from build123d import *


with BuildPart() as part:
    # Sketch2 → Revolve1 (revolve)
    with BuildSketch(Plane.XY, mode=Mode.PRIVATE) as revolve1_sk:
        with BuildLine():
            Line((7.900124766, 45.904993762), (46, 44))
            Line((46, 44), (46, 40))
            Line((46, 40), (8, 40))
            ThreePointArc((8, 40), (6.585786438, 39.414213562), (6, 38))
            Line((6, 38), (6, 2))
            Line((6, 2), (0, 2))
            Line((0, 2), (0, 76.2))
            Line((0, 76.2), (6.299212598, 76.2))
            Line((6.299212598, 76.2), (100, 76.2))
            Line((100, 76.2), (100, 73.2))
            Line((100, 73.2), (8, 73.2))
            ThreePointArc((8, 73.2), (6.585786438, 72.614213562), (6, 71.2))
            Line((6, 71.2), (6, 47.902498439))
            ThreePointArc((6, 47.902498439), (6.550905374, 46.524048308), (7.900124766, 45.904993762))
        make_face()
    revolve(revolve1_sk.sketch.rotate(Axis((0, 0, 0), (1, 0, 0)), 90), axis=Axis((0, 0, 0), (1, 0, 0)))


solid = part.part
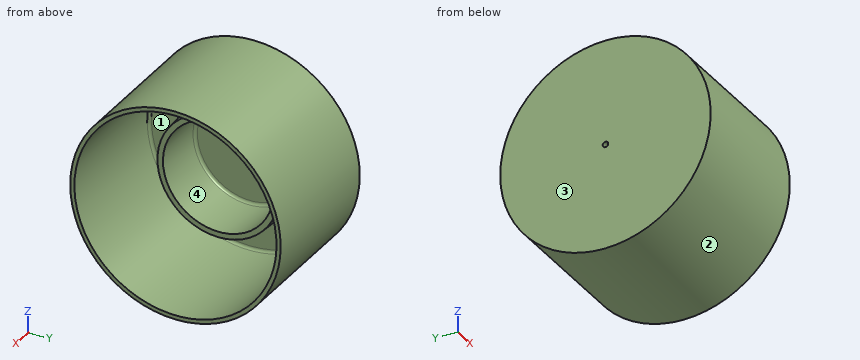
Input: part model. Units: mm. Frame: model coordinates. Face numbers are marked on the shaded views. Give positions to 0.01 mm unless a question says otherwise; leave off trailing zeros. Order: outer loops, then holes, each group sorted by start corner. A loop starts at its lowest first (then second) coordinate and runs counter-clockwise, first axis right, second up. Notation, with made-up numbers: M 80,14.5 L 128,14.5 A37 ccw 128,50.5 Z; hole C 62.25,9.25 d3. An arc over 180 degrees is marked long. Answer as a JSON object with one key per item and string values.
1. Cut plane B-B, the plane x = 22. Output: boundary loops of the cut face in (y, z).
Result sheet:
{"outline": "C 0,0 d152.4; C 0,0 d90.4; hole C 0,0 d146.4; hole C 0,0 d80"}
2. Cut plane D-D, the plane x = 41. Output: boundary loops of the cut face in (y, z), and give its area (3 significant figures).
Result sheet:
{"outline": "C 0,0 d152.4; C 0,0 d88.5; hole C 0,0 d146.4; hole C 0,0 d80", "area": "2,530 mm²"}
3. Ray query, line 1 (Y direction, x = 3.7, z = 0); line 2 (Y direction, x = 26, z = -8); line 3 (Y direction, x = 43, z = 0). Return the intervals inside material, ascending. Write a range as [from, to].
Result sheet:
{"line 1": "[-76.2, -2], [2, 76.2]", "line 2": "[-75.78, -72.76], [-44.28, -39.19], [39.19, 44.28], [72.76, 75.78]", "line 3": "[-76.2, -73.2], [-44.15, -40], [40, 44.15], [73.2, 76.2]"}
4. Cut plane A-A, the plane z = 0. Output: boundary loops of the cut face in (x, y) (1 decimal).
Result sheet:
{"outline": "M 0,-76.2 L 100,-76.2 L 100,-73.2 L 8,-73.2 A2 cw 6,-71.2 L 6,-47.9 A2 cw 7.9,-45.9 L 46,-44 L 46,-40 L 8,-40 A2 cw 6,-38 L 6,-2 L 0,-2 Z; M 0,2 L 6,2 L 6,38 A2 cw 8,40 L 46,40 L 46,44 L 7.9,45.9 A2 cw 6,47.9 L 6,71.2 A2 cw 8,73.2 L 100,73.2 L 100,76.2 L 0,76.2 Z"}
5. Pull-direction query (Y, two-part tool) for the marked faces 1, 2, 3 and 4; classes: +Y half, -Y half, draft (parallel to the pull), parting line (faces both ways), or undercut.
Result sheet:
{"face 1": "undercut", "face 2": "parting line", "face 3": "draft", "face 4": "undercut"}
6. First-contact query: P1, Ø8, axis at x = 44, z = 21, coming from the -Y side; P2, Ø2, axis at x = 46.5, z = 10.5, coming from the +Y side; P3, Ø6, axis at x = 82, y = -46.5, coming from the -Z side. Flat tips, straight axial feed; report the tip coordinate or a pass-through.
Result sheet:
{"P1": "y = -74.28", "P2": "y = 75.61", "P3": "z = -62.56"}
